```python
from build123d import *

# Parameters (mm, degrees)
SKETCH1_W           = 70
SKETCH1_H           = 160
BOSS_EXTRUDE1_DEPTH = 3
SKETCH2_W           = 20
SKETCH2_H           = 3
CUT_EXTRUDE1_DEPTH  = 3
SKETCH3_W           = 3
SKETCH3_H           = 20
BOSS_EXTRUDE2_DEPTH = 3
SKETCH5_W           = 40
SKETCH5_H           = 65
CUT_EXTRUDE2_DEPTH  = 25


with BuildPart() as part:
    # Sketch1 → Boss-Extrude1 (new body)
    with BuildSketch(Plane(origin=(0, 0, 0), x_dir=(1, 0, 0), z_dir=(0, 1, 0))):
        with Locations((35, 80)):
            Rectangle(SKETCH1_W, SKETCH1_H)
    extrude(amount=BOSS_EXTRUDE1_DEPTH)

    # Sketch2 → Cut-Extrude1 (cut)
    with BuildSketch(Plane(origin=(0, 3, 0), x_dir=(1, 0, 0), z_dir=(0, 1, 0))):
        with Locations((10, 28.5)):
            Rectangle(SKETCH2_W, SKETCH2_H)
        with Locations((10, 131.5)):
            Rectangle(SKETCH2_W, SKETCH2_H)
        with Locations((50, 131.5)):
            Rectangle(SKETCH2_W, SKETCH2_H)
        with Locations((50, 28.5)):
            Rectangle(SKETCH2_W, SKETCH2_H)
    extrude(amount=-CUT_EXTRUDE1_DEPTH, mode=Mode.SUBTRACT)

    # Sketch3 → Boss-Extrude2 (add)
    with BuildSketch(Plane(origin=(0, 3, 0), x_dir=(1, 0, 0), z_dir=(0, 1, 0))):
        with Locations((-1.5, 120)):
            Rectangle(SKETCH3_W, SKETCH3_H)
        with Locations((-1.5, 80)):
            Rectangle(SKETCH3_W, SKETCH3_H)
        with Locations((-1.5, 40)):
            Rectangle(SKETCH3_W, SKETCH3_H)
    extrude(amount=-BOSS_EXTRUDE2_DEPTH)

    # Sketch5 → Cut-Extrude2 (cut)
    with BuildSketch(Plane(origin=(0, 3, 0), x_dir=(1, 0, 0), z_dir=(0, 1, 0))):
        with Locations((50, 80)):
            Rectangle(SKETCH5_W, SKETCH5_H)
    extrude(amount=-CUT_EXTRUDE2_DEPTH, mode=Mode.SUBTRACT)


solid = part.part
```
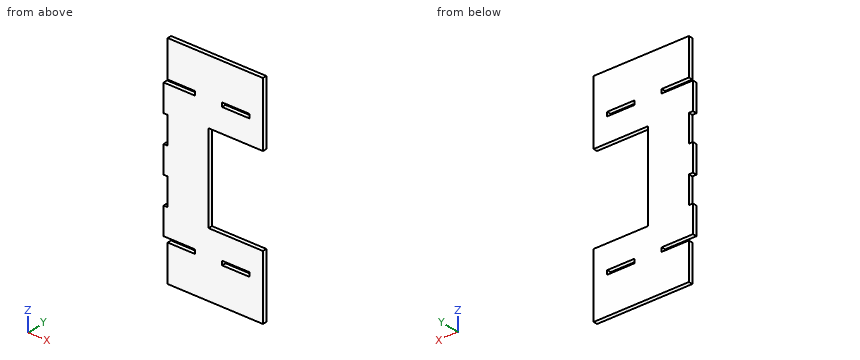
Input: part model. Units: mm. Frame: model coordinates. Give positions to 0.01 mm unless a question says otherwise; leave off trailing zeros. Order: outer loops, then holes, each group sorted by start corner. A loop starts at its lowest first (then second) coordinate and runs counter-clockwise, first axis right, second up. Notation, with made-up numbers: (7.25, 49) - (34.25, 49) arc R31 cw to (34.25, 81) - close; hole circle Ø11 at (-33.75, 25.25). An arc over 180 degrees is marked (long way). Put each result on its own line as item: value.
Item 1: Section query A-A, the plane x = 32. Return loops of the section in (y, z).
Found:
outline: (0, -160) - (3, -160) - (3, -112.5) - (0, -112.5) - close; (0, -47.5) - (3, -47.5) - (3, 0) - (0, 0) - close
Item 2: Contact query for flat-ended pins moving along their axis: pin 1 (0.9 mm diameter, centred on y = 1.5, z = -131.5, fed in from -X); pin 2 (1 mm diameter, centred on y = 1, z = -17.5, fed in from -X). Output: stop coordinate, or through.
Found:
pin 1: stops at x = 20
pin 2: stops at x = 0
Item 3: Section query B-B, the plane x = 16.5. Return loops of the section in (y, z).
Found:
outline: (0, -160) - (3, -160) - (3, -133) - (0, -133) - close; (0, -130) - (3, -130) - (3, -30) - (0, -30) - close; (0, -27) - (3, -27) - (3, 0) - (0, 0) - close
Item 4: Section query D-D, the plane z = -131.5. Return loops of the section in (x, y), then the cut area to 3 significant figures.
Found:
outline: (20, 0) - (40, 0) - (40, 3) - (20, 3) - close; (60, 0) - (70, 0) - (70, 3) - (60, 3) - close
area: 90.0 mm^2
Item 5: Section query C-C, the plane y = 1.1. Count the separate pieces of the cut face and the enclosed holes in it, then the cut area to 3 significant figures.
Found:
separate pieces: 1
enclosed holes: 2
area: 8,540 mm^2
Item 6: Ray query, L1, parallel to Z at x = 55.5, y = 1.65; L2, parallel to Z at x = 18, y = 2.4; L3, parallel to X at y = 2.85, z = -132.5. Return the intervals inside material, ascending. Write a range as from..to.
Found:
L1: z = -160..-133, -130..-112.5, -47.5..-30, -27..0
L2: z = -160..-133, -130..-30, -27..0
L3: x = 20..40, 60..70
